Build history of the part. All positions in model axes, mm. Face numbers are marked on the shaded views. A direction names the side the tool comes from. Give positions to 0.01 mm unless a question says otherwise; leave off trailing zeros. Order: outer loops, then holes, each group sorted by start corner. A loop starts at its lowest first (then second) coordinate and runs counter-clockwise, first axis right, second up. Notation, with made-up numbers: (76.25, 68.25) - (98.25, 68.25) arc R28 cw to (98.25, 94.25) - close; hole circle Ø3 at (3.25, -13.75). An arc over 180 degrees is marked (long way). Use a Markdown table: item, result.
from build123d import *

# Parameters (mm, degrees)
BOSS_EXTRUDE1_DEPTH      = 5
SKETCH2_3_R              = 19
SKETCH2_3_R_2            = 10
BOSS_EXTRUDE2_DEPTH      = 15
SKETCH2_5_R              = 32
SKETCH2_5_R_2            = 27.5
BOSS_EXTRUDE3_DEPTH      = 15
BOSS_EXTRUDE4_DEPTH      = 30
BOSS_EXTRUDE4_DEPTH_BACK = 15
SKETCH2_6_R              = 21.5
SKETCH2_6_R_2            = 17
SKETCH2_7_R              = 27.5
SKETCH2_7_R_2            = 21.5
BOSS_EXTRUDE5_DEPTH      = 12.5


with BuildPart() as part:
    # Sketch2 → Boss-Extrude1 (new, symmetric)
    with BuildSketch(Plane.XY):
        with BuildLine():
            ThreePointArc((-18.724325041, 17.664638492), (7.753239465, 31.999343197), (34.412311606, 18.005092456))
            ThreePointArc((34.412311606, 18.005092456), (24.526384504, 42.934747234), (26.204222758, 69.700473468))
            ThreePointArc((26.204222758, 69.700473468), (7.817165129, 56.000523924), (-10.364391673, 69.972048465))
            ThreePointArc((-10.364391673, 69.972048465), (-8.883681263, 42.913636414), (-18.724325041, 17.664638492))
        make_face()
    extrude(amount=BOSS_EXTRUDE1_DEPTH, both=True)

    # Sketch2<3> → Boss-Extrude2 (add, symmetric)
    with BuildSketch(Plane.XY):
        with Locations((7.958263794, 75)):
            Circle(SKETCH2_3_R)
        with Locations((7.958263794, 75)):
            Circle(SKETCH2_3_R_2, mode=Mode.SUBTRACT)
    extrude(amount=BOSS_EXTRUDE2_DEPTH, both=True)

    # Sketch2<5> → Boss-Extrude3 (add, symmetric)
    with BuildSketch(Plane.XY):
        with Locations((7.958263794, 0)):
            Circle(SKETCH2_5_R)
        with Locations((7.958263794, 0)):
            Circle(SKETCH2_5_R_2, mode=Mode.SUBTRACT)
    extrude(amount=BOSS_EXTRUDE3_DEPTH, both=True)



with BuildPart() as body_2:
    # Sketch2<6> → Boss-Extrude4 (new, two sides: drawn at the far end of the back side and taken through both)
    with BuildSketch(Plane.XY.offset(-BOSS_EXTRUDE4_DEPTH_BACK)):
        with Locations((7.958263794, 0)):
            Circle(SKETCH2_6_R)
        with Locations((7.958263794, 0)):
            Circle(SKETCH2_6_R_2, mode=Mode.SUBTRACT)
    extrude(amount=BOSS_EXTRUDE4_DEPTH + BOSS_EXTRUDE4_DEPTH_BACK)


with BuildPart() as part_1:
    add(part.part)

    add(body_2.part)  # Boss-Extrude5 merges body 2
    # Sketch2<7> → Boss-Extrude5 (add, symmetric)
    with BuildSketch(Plane.XY):
        with Locations((7.958263794, 0)):
            Circle(SKETCH2_7_R)
        with Locations((7.958263794, 0)):
            Circle(SKETCH2_7_R_2, mode=Mode.SUBTRACT)
    extrude(amount=BOSS_EXTRUDE5_DEPTH, both=True)


solid = part_1.part
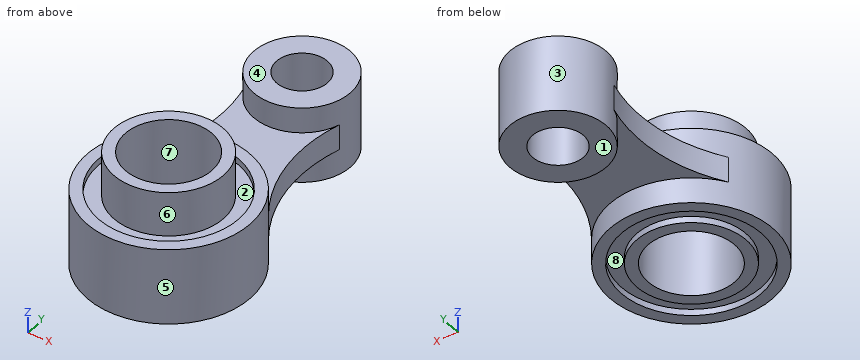
1) Slice it at C-C (z = -8). Write the cut outline in (x, y), and give its area (3 significant figures).
Computed:
| item | result |
|---|---|
| outline | circle Ø64 at (7.96, 0); circle Ø38 at (7.96, 75); hole circle Ø34 at (7.96, 0); hole circle Ø20 at (7.96, 75) |
| area | 3,130 mm² |
2) Two-plate mould, pull along X, no slides. Class the marked faces 1, 2 and 3: +X half, -X half, draft (parallel to the pull), parting line (faces both ways), or undercut.
Computed:
| item | result |
|---|---|
| face 1 | draft |
| face 2 | undercut |
| face 3 | parting line |
3) Wall check: line 1 (Y direction, x = 7.5, z = 5.5); line 2 (Y direction, x = 0, z = -7); line 3 (X direction, y = 4.5, z = -0.5). Give the ranges that are in metal, low to high. Write a range as from..to.
Computed:
| item | result |
|---|---|
| line 1 | y = -32..-16.99, 16.99..32, 56.01..65.01, 84.99..93.99 |
| line 2 | y = -30.99..-15.02, 15.02..30.99, 57.75..68.94, 81.06..92.25 |
| line 3 | x = -23.72..-8.44, 24.35..39.64 |
4) Pin check, flat tips, straight feed: P1, Ø10, axis at x = -5, y = 74, coming from the +Z side; P2, Ø4, axis at x = -11.5, y = 65.5, coming from the +Z side; P3, Ø4, axis at x = -11.5, z = 25, coming from the -Y side; P4, Ø2, axis at x = 32, y = -5.5, coming from the +Z side. Stop position of each tip, or through.
Computed:
| item | result |
|---|---|
| P1 | stops at z = 15 |
| P2 | passes through |
| P3 | stops at y = -12.55 |
| P4 | stops at z = 12.5 |
5) Tool access for the marked faces 4, 5, 6, 7 and 8: list every direction of +Z, -Z, +X, -X, +Y, -Y with a clear straight run to the whole face (end or side of a thin tool).
Computed:
| item | result |
|---|---|
| face 4 | +Z, +X, -X, +Y |
| face 5 | none |
| face 6 | +Z |
| face 7 | +Z, -Z |
| face 8 | -Z |
6) Slice it at A-A (y = 0). Write the cut outline in (x, z), and give its area (3 significant figures).
Computed:
| item | result |
|---|---|
| outline | (-24.04, -15) - (-19.54, -15) - (-19.54, -12.5) - (-13.54, -12.5) - (-13.54, -15) - (-9.04, -15) - (-9.04, 30) - (-13.54, 30) - (-13.54, 12.5) - (-19.54, 12.5) - (-19.54, 15) - (-24.04, 15) - close; (24.96, -15) - (29.46, -15) - (29.46, -12.5) - (35.46, -12.5) - (35.46, -15) - (39.96, -15) - (39.96, 15) - (35.46, 15) - (35.46, 12.5) - (29.46, 12.5) - (29.46, 30) - (24.96, 30) - close |
| area | 975 mm² |
7) Slice it at D-D (y = 75). Write the cut outline in (x, z), and give its area (3 significant figures).
Computed:
| item | result |
|---|---|
| outline | (-11.04, -15) - (-2.04, -15) - (-2.04, 15) - (-11.04, 15) - close; (17.96, -15) - (26.96, -15) - (26.96, 15) - (17.96, 15) - close |
| area | 540 mm² |
